Work out the finished part from the listing and answer in its coordinate system (mm). A direction names the side the tool comes from. Coordinates: 2 decimals unless noted, no trailing zeros. Loops run counter-clockwise (first coordinate to the right, second up) from the corner with the lowest first, then second, coordinate; pieces in that order, holes last. Notation, with made-up numbers: (17.5, -16) -> (23.5, -16) arc R27 cw to (23.5, 23) -> close; hole circle Ø10 at (20.5, 36). An arc over 180 degrees is marked (long way). Answer as CSV lines item,"result".
```python
from build123d import *

# Parameters (mm, degrees)
F0_R     = 19.05
F1_DEPTH = 31.75
F2_R     = 5.5626
F3_DEPTH = 4.7752
F4_DEPTH = 57.151


with BuildPart() as f1:
    # F0 (on Front) → F1 (new body, symmetric)
    with BuildSketch(Plane.XZ):
        with BuildLine():
            Line((139.5674778593, 28.575), (0, 28.575))
            ThreePointArc((0, 28.575), (-19.345366451, -21.0306305629), (28.4756083945, 2.38125))
            ThreePointArc((28.4756083945, 2.38125), (30.9572676717, 9.6234554837), (37.9674778593, 12.7))
            Line((37.9674778593, 12.7), (139.5674778593, 12.7))
            Line((139.5674778593, 12.7), (139.5674778593, 28.575))
        make_face()
        Circle(F0_R, mode=Mode.SUBTRACT)
    extrude(amount=F1_DEPTH, both=True)

    # F2 (on face) → F3 (join)
    with BuildSketch(Plane.XY.offset(28.575)):
        with BuildLine():
            ThreePointArc((56.9407035424, 30.1667333333), (44.3462001498, 29.9879370767), (38.1, 19.05))
            Line((38.1, 19.05), (38.1, -19.05))
            ThreePointArc((38.1, -19.05), (44.5021137711, -30.078446357), (57.2537998502, -29.9879370767))
            Line((57.2537998502, -29.9879370767), (90.6039998502, -10.3100477039))
            ThreePointArc((90.6039998502, -10.3100477039), (96.8489204336, 0.8081651333), (90.2909035424, 11.7446227062))
            Line((90.2909035424, 11.7446227062), (56.9407035424, 30.1667333333))
        make_face()
        with Locations((50.8, -19.05)):
            Circle(F2_R, mode=Mode.SUBTRACT)
        with Locations((50.8, 19.05)):
            Circle(F2_R, mode=Mode.SUBTRACT)
        with Locations((84.1502, 0.6278893728)):
            Circle(F2_R, mode=Mode.SUBTRACT)
    extrude(amount=F3_DEPTH)

    # F4 (cut, through all): faces of the model
    f4_faces = [f1.faces().sort_by_distance(p)[0] for p in [
        (50.8, 19.05, 28.575),
        (84.1502, 0.6278893728, 28.575),
        (50.8, -19.05, 28.575),
        (108.2569186548, -0.1131496347, 28.575),
    ]]
    extrude(f4_faces, amount=-F4_DEPTH, mode=Mode.SUBTRACT)


solid = f1.part
```
(1) A cutting plane is placed at C-C, the plane y = 17. Write down the section's boundary in (x, z) (3 decimals).
Computed values:
outline,"(0, 28.575) arc R28.575 ccw (long way) to (28.476, 2.381) arc R9.525 cw to (37.967, 12.7) -> (45.629, 12.7) -> (45.629, 33.35) -> (38.1, 33.35) -> (38.1, 28.575) -> close; (55.971, 12.7) -> (80.777, 12.7) -> (80.777, 33.35) -> (55.971, 33.35) -> close; hole circle Ø38.1 at (0, 0)"
(2) Flat-ended cylindrical pins translate along their axes: pin 1 Ø14.5 at (x, y) = (50.8, -19.05) entering from -Z; pin 2 Ø3 at (x, y) = (15, 23.5) entering from -Z; pin 3 Ø4 at (y, z) = (20.5, 11.5) entering from -X. Find the tip coordinate at first contact, or state that the pin passes through.
Computed values:
pin 1,"z = 12.7"
pin 2,"z = -25.18"
pin 3,"x = -26.95"
(3) A cutting plane is placed at A-A, the plane z = 0. Write down the section's boundary in (x, y) (3 decimals), and give its area (3 significant figures).
Computed values:
outline,"(-28.575, -31.75) -> (-19.05, -31.75) -> (-19.05, 31.75) -> (-28.575, 31.75) -> close; (19.05, -31.75) -> (28.575, -31.75) -> (28.575, 31.75) -> (19.05, 31.75) -> close"
area,"1,210 mm2"
(4) Consider line 1 along X through (y, z) = (14, 17.5); line 2 along X through (y, z) = (4, 13.5); line 3 along Y through (x, z) = (47, 16.5). Determine where each line is inside the solid, lowest interval first.
Computed values:
line 1,"-22.59 to -7.53, 7.53 to 48.47, 53.13 to 86.21"
line 2,"-25.18 to -13.44, 13.44 to 79.73, 88.57 to 96.39"
line 3,"-31.75 to -23.11, -14.99 to 14.99, 23.11 to 31.75"
(5) For a pull along X with two mould halves and no side action, classify faces 4 (the face through (38.1, 0, 31)), 5 (the face through (50.07, 31.73, 29.76)), 6 (the face through (-15.12, 0.44, -11.59)), 7 (the face through (19, 31.75, 7)) as pulls with the +X half, pulls with the -X half, needs draft (parallel to the pull), parting line crosses it, or undercut.
Computed values:
face 4,"pulls with the -X half"
face 5,"parting line crosses it"
face 6,"undercut"
face 7,"needs draft"
(6) A cutting plane is placed at D-D, the plane y = 7.5. Write down the section's boundary in (x, z) (3 decimals), and give its area (3 significant figures).
Computed values:
outline,"(0, 28.575) arc R28.575 ccw (long way) to (28.476, 2.381) arc R9.525 cw to (37.967, 12.7) -> (94.83, 12.7) -> (94.83, 33.35) -> (38.1, 33.35) -> (38.1, 28.575) -> close; hole circle Ø38.1 at (0, 0)"
area,"2,940 mm2"
(7) Which of the six approach directions +Z, -Z, +X, -X, +Y, -Y give full straight-line access (tool end or side, diameter ignored) to faces 1 (the face through (49.962, -31.722, 29.764)), 2 (the face through (73.695, -20.287, 22.881)), 3 (the face through (60, 0, 12.7))?
Computed values:
face 1,"+Z, -Y"
face 2,"+Z, -Z, +X, -Y"
face 3,"-Z, +X, +Y, -Y"
(8) A cutting plane is placed at B-B, the plane x = 7. Write down the section's boundary in (y, z) (3 decimals).
Computed values:
outline,"(-31.75, -27.704) -> (31.75, -27.704) -> (31.75, -17.717) -> (-31.75, -17.717) -> close; (-31.75, 17.717) -> (31.75, 17.717) -> (31.75, 28.575) -> (-31.75, 28.575) -> close"
